```python
from build123d import *

# Parameters (mm, degrees)
SKIZZE1_R                       = 2.5
AUFSATZ_LINEAR_AUSTRAGEN1_DEPTH = 2
SKIZZE2_R                       = 1
AUFSATZ_LINEAR_AUSTRAGEN2_DEPTH = 8
VERRUNDUNG1_R                   = 1


with BuildPart() as part:
    # Skizze1 → Aufsatz-Linear austragen1 (new body)
    with BuildSketch(Plane(origin=(0, 0, 0), x_dir=(0, 0, -1), z_dir=(1, 0, 0))):
        Circle(SKIZZE1_R)
    extrude(amount=AUFSATZ_LINEAR_AUSTRAGEN1_DEPTH)

    # Skizze2 → Aufsatz-Linear austragen2 (add)
    with BuildSketch(Plane.ZY):
        Circle(SKIZZE2_R)
    extrude(amount=AUFSATZ_LINEAR_AUSTRAGEN2_DEPTH)

    # Verrundung1
    verrundung1_edges = [part.edges().sort_by_distance(p)[0] for p in [
        (2, 0, 2.5),
    ]]
    fillet(verrundung1_edges, radius=VERRUNDUNG1_R)


solid = part.part
```
Verification items for the finished model (mm, model axes). A direction names the side the tool comes from. Round coordinates to 2 decimals unless told otherwise and drop trailing zeros. Write each loop counter-clockwise with the first axis right and the second up, starting at its lowest first coordinate (ties: lowest second). Pieces come first, ordered by that corner, then holes. Notation, with made-up numbers: (20, 40) - (64, 40) arc R34 ccw to (64, 74) - close; hole circle Ø10 at (49.5, 1.25). An arc over 180 degrees is marked (long way). Answer as a JSON object with one key per item and string values. Group by question number.
Q1. Thickness scan on line 1 (X direction, y = -0.15, z = 1.2); line 2 (Y direction, x = -7.25, z = -0.75); line 3 (Y direction, x = -6.75, z = -0.05). Record the ranges inside material, lowest first.
Q2. Tool access check on faces 3 (the cylindrical face through (-4, -1, 0)), 4 (the flat face through (2, 0, 0)). Record the directions out of +Z, -Z, +X, -X, +Y, -Y that give a thin tool (end or side, any length) a straight path to the whole face; none if there is none.
Q3. Mould release check, pull along Y, two halves, no side actions. Record for faces 1 (the cylindrical face through (0.49, -2.44, 0.54)), 2 (the flat face through (-8, 0, 0)): released by +Y, released by -Y, zero draft, split by the parting line, or undercut.
Q4. Section check A-A, the plane y = 0. Enter the section's corners in (x, z).
Q5. Section check C-C, the plane x = -4.5. Enter the section's corners in (y, z), plus the area to 3 significant figures.
Q6. Section check D-D, the plane x = 1.75. Enter the section's corners in (y, z).
Found:
{
 "1": {"line 1": "x = 0 to 2", "line 2": "y = -0.66 to 0.66", "line 3": "y = -1 to 1"},
 "2": {"face 3": "-X", "face 4": "+Z, -Z, +X, +Y, -Y"},
 "3": {"face 1": "split by the parting line", "face 2": "zero draft"},
 "4": {"outline": "(-8, -1) - (0, -1) - (0, -2.5) - (1, -2.5) arc R1 ccw to (2, -1.5) - (2, 1.5) arc R1 ccw to (1, 2.5) - (0, 2.5) - (0, 1) - (-8, 1) - close"},
 "5": {"outline": "circle Ø2 at (0, 0)", "area": "3.14 mm^2"},
 "6": {"outline": "circle Ø4.32 at (0, 0)"}
}
